```python
from build123d import *

# Parameters (mm, degrees)
SKETCH_1_R          = 11
EXTRUDE_1_DEPTH     = 5
SKETCH_1_R_2        = 6
EXTRUDE_1_2_DEPTH   = 5
EXTRUDE_3_DEPTH     = 5
SKETCH_4_R          = 11.25
CUT_EXTRUDE_1_DEPTH = 2.5
SKETCH_5_R          = 5
CUT_EXTRUDE_2_DEPTH = 6
SKETCH_6_R          = 4
SKETCH_6_R_2        = 2.5
CUT_EXTRUDE_3_DEPTH = 6
CUT_EXTRUDE_4_DEPTH = 6
SKETCH_8_R          = 0.747737987
SKETCH_8_R_2        = 0.75
CUT_EXTRUDE_5_DEPTH = 3.5
SKETCH_9_R          = 4.25
CUT_EXTRUDE_6_DEPTH = 3.5


with BuildPart() as part:
    # Sketch 1 → Extrude 1 (new body)
    with BuildSketch(Plane(origin=(0, 0, 0), x_dir=(1, 0, 0), z_dir=(0, 1, 0))):
        with Locations((-44.318784969, 0)):
            Circle(SKETCH_1_R)
    extrude(amount=EXTRUDE_1_DEPTH)



with BuildPart() as body_2:
    # Sketch 1 → Extrude 1 2 (new body)
    with BuildSketch(Plane(origin=(0, 0, 0), x_dir=(1, 0, 0), z_dir=(0, 1, 0))):
        with Locations((35.681215031, 0)):
            Circle(SKETCH_1_R_2)
    extrude(amount=EXTRUDE_1_2_DEPTH)


with BuildPart() as part_1:
    add(part.part)

    add(body_2.part)  # Extrude 3 merges body 2
    # Sketch 3 → Extrude 3 (add)
    with BuildSketch(Plane(origin=(0, 0, 0), x_dir=(1, 0, 0), z_dir=(0, 1, 0))):
        Polygon((-44.318784969, 11), (35.681215031, 6), (35.681215031, -6), (-44.318784969, -11), align=None)
    extrude(amount=EXTRUDE_3_DEPTH)

    # Sketch 4 → Cut-Extrude 1 (cut)
    with BuildSketch(Plane(origin=(0, 5, 0), x_dir=(1, 0, 0), z_dir=(0, 1, 0))):
        with Locations((-44.318784969, 0)):
            Circle(SKETCH_4_R)
    extrude(amount=-CUT_EXTRUDE_1_DEPTH, mode=Mode.SUBTRACT)

    # Sketch 5 → Cut-Extrude 2 (cut, through all)
    with BuildSketch(Plane(origin=(0, 5, 0), x_dir=(1, 0, 0), z_dir=(0, 1, 0))):
        with Locations((35.681215031, 0)):
            Circle(SKETCH_5_R)
    extrude(amount=-CUT_EXTRUDE_2_DEPTH, mode=Mode.SUBTRACT)

    # Sketch 6 → Cut-Extrude 3 (cut, through all)
    with BuildSketch(Plane(origin=(0, 5, 0), x_dir=(1, 0, 0), z_dir=(0, 1, 0))):
        with Locations((-22, 0)):
            Circle(SKETCH_6_R)
        with Locations((18, 0)):
            Circle(SKETCH_6_R_2)
    extrude(amount=-CUT_EXTRUDE_3_DEPTH, mode=Mode.SUBTRACT)

    # Sketch 7 → Cut-Extrude 4 (cut, through all)
    with BuildSketch(Plane(origin=(0, 5, 0), x_dir=(1, 0, 0), z_dir=(0, 1, 0))):
        Polygon((-22, 4), (18, 2.5), (18, -2.5), (-22, -4), align=None)
    extrude(amount=-CUT_EXTRUDE_4_DEPTH, mode=Mode.SUBTRACT)

    # Sketch 8 → Cut-Extrude 5 (cut, through all)
    with BuildSketch(Plane(origin=(0, 2.5, 0), x_dir=(1, 0, 0), z_dir=(0, 1, 0))):
        with Locations((-52.318784969, 0)):
            Circle(SKETCH_8_R)
        with Locations((-36.318784969, 0)):
            Circle(SKETCH_8_R)
        with Locations((-44.318784969, 8)):
            Circle(SKETCH_8_R_2)
        with Locations((-44.318784969, -8)):
            Circle(SKETCH_8_R_2)
    extrude(amount=-CUT_EXTRUDE_5_DEPTH, mode=Mode.SUBTRACT)

    # Sketch 9 → Cut-Extrude 6 (cut, through all)
    with BuildSketch(Plane(origin=(0, 2.5, 0), x_dir=(1, 0, 0), z_dir=(0, 1, 0))):
        with Locations((-44.318784969, 0)):
            Circle(SKETCH_9_R)
    extrude(amount=-CUT_EXTRUDE_6_DEPTH, mode=Mode.SUBTRACT)


solid = part_1.part
```
The model under review builds one solid part; all positions refer to its coordinate system, in mm. A direction names the side the tool comes from. Round coordinates to 2 decimals unless told otherwise and drop trailing zeros. Write each loop counter-clockwise with the first axis right and the second up, starting at its lowest first coordinate (ties: lowest second). Pieces come first, ordered by that corner, then holes. Notation, with made-up numbers: (-17.75, -35) - (-1.75, -35) arc R23 ccw to (-1.75, -5) - close; hole circle Ø10 at (-26, 60.25). An arc over 180 degrees is marked (long way). Answer as CSV lines item,"result". Start each with the question number.
(1) We need section A-A on y = 3.35. State the section outline as (x, z) points, plus the area to 3 significant figures.
(2) Draft analysis for pull direction Z (two halves, no side actions). For faces 1 (the cylindrical face through (-53.066, 1.268, -0.033)), 2 (the cylindrical face through (-55.316, 1.232, -0.261)), 3 (the flat face through (-18, 0, 5)), state which applies: pulls with the +Z half, pulls with the -Z half, needs draft (parallel to the pull), parting line crosses it, or undercut.
(3) To check wall thickness, follow line 1 (X direction, y = 0.7, z = 0); line 2 (X direction, y = 3, z = 2); line 3 (X direction, y = 4.2, z = 0.25). State the ranges of each line that lie inside material, in increasing order.
(4) We need section C-C on x = -5. State the section outline as (y, z) points, plus the area to 3 significant figures.
(5) For pin 1 Ø4 at (x, z) = (-38.5, 4) entering from +Y; pin 2 Ø1.5 at (y, z) = (1, -1.5) entering from -X, all flat-tipped, find the tip position at first contact; note any pin that passes through.
(6) We need section D-D on x = 27.5. State the section outline as (y, z) points.
(7) We need section B-B on x = -46.5. State the section outline as (y, z) points.
(8) For faces 4 (the flat face through (-44, 2.5, 5)), 5 (the cylindrical face through (20.5, 2.5, 0.1)), 6 (the flat face through (-3.084, 2.465, 8.423)), list the 3-axis set-ups (+Z, -Z, +X, -X, +Y, -Y) from which the entire face can be reached by the end or side of a thin tool; tool diameter is ignored.
Worked answers:
1,outline,"(-41.18, -10.8) - (35.68, -6) arc R6 ccw to (35.68, 6) - (-41.18, 10.8) arc R11.25 cw to start; hole (-21.7, -3.99) - (18, -2.5) arc R2.5 ccw to (18, 2.5) - (-21.7, 3.99) arc R4 ccw (long way) to start; hole circle Ø10 at (35.68, 0)"
1,area,"846 mm²"
2,face 1,"undercut"
2,face 2,"parting line crosses it"
2,face 3,"needs draft"
3,line 1,"-55.32 to -53.07, -51.57 to -48.57, -40.07 to -37.07, -35.57 to -26, 20.5 to 30.68, 40.68 to 41.68"
3,line 2,"-33.25 to -25.46, 19.5 to 31.1, 40.26 to 41.34"
3,line 3,"-33.07 to -25.99, 20.49 to 30.69, 40.67 to 41.68"
4,outline,"(0, -8.54) - (5, -8.54) - (5, -3.36) - (0, -3.36) - close; (0, 3.36) - (5, 3.36) - (5, 8.54) - (0, 8.54) - close"
4,area,"51.8 mm²"
5,pin 1,"y = 2.5"
5,pin 2,"x = -55.29"
6,outline,"(0, -6.51) - (5, -6.51) - (5, 6.51) - (0, 6.51) - close"
7,outline,"(0, -10.78) - (2.5, -10.78) - (2.5, -3.65) - (0, -3.65) - close; (0, 3.65) - (2.5, 3.65) - (2.5, 10.78) - (0, 10.78) - close"
8,face 4,"-X, +Y"
8,face 5,"+Y, -Y"
8,face 6,"+Z, +X, +Y, -Y"
